Work out the finished part from the listing and answer in its coordinate system (mm). A direction names the side the tool comes from. Give positions to 0.01 mm unless a question says otherwise; leave off trailing zeros. Order: outer loops, then holes, each group sorted by start corner. A loop starts at its lowest first (then second) coordinate and runs counter-clockwise, first axis right, second up. Notation, with made-up numbers: (39.5, 44.25) -> (63.5, 44.25) arc R16 cw to (63.5, 65.25) -> close; hole circle Ø4 at (-19, 84.25). An arc over 180 degrees is marked (long way). Answer as CSV lines item,"result". Start each with the question number.
1. Find the intervals of material crossed by L1, parallel to X at y = 7.2, z = 0; L2, parallel to Z at x = -10.5, y = 13.25; L3, parallel to Y at x = -14.5, z = -18, in increasing order.
2. A cutting plane is placed at A-A (y = 6). Give the vertices of the cut face in (x, z).
3. A cutting plane is placed at B-B (x = 0). Give the vertices of the cut face in (y, z).
4. Flat-ended cylindrical pins translate along their axes: pin 1 (0.7 mm diameter, centred on y = 11.5, z = 3.5, fed in from +X); pin 2 (6 mm diameter, centred on x = -10, y = 17, fed in from -Z); pin 3 (7 mm diameter, centred on x = 0, z = 0, fed in from +Y). Find the tip coordinate at first contact, or state that the pin passes through.
5. A cutting plane is placed at D-D (x = -44). Give the vertices of the cut face in (y, z), then the cut area to 3 significant figures.
6. For faces 1 (the flat face through (-56.2, 18.7, 4.4)), 2 (the flat face through (-64.507, 18.803, -43.287)), 3 (the flat face through (-64, 16, -51.985)), determine the directions among +Z, -Z, +X, -X, +Y, -Y from which every point of the face is accessible in a straight line to the end or side of a thin tool.
7. For a pull along Z with two mould halves and no side action, classify faces 4 (the flat face through (-52.5, 12, 4)), 5 (the flat face through (-56.67, 18.45, 3.29)), 6 (the flat face through (-64, 12, -7.5)) as released by +Z, released by -Z, zero draft, split by the parting line, or undercut.
8. A cutting plane is placed at C-C (z = -56.5). Give the vertices of the cut face in (x, y), then the cut area to 3 significant figures.
from build123d import *

# Parameters (mm, degrees)
SKETCH1_W           = 10.000000000000004
SKETCH1_H           = 10
SKETCH1_W_2         = 10
BOSS_EXTRUDE1_DEPTH = 10
SKETCH2_W           = 1.999999999999993
SKETCH2_H           = 10.29963091051744
SKETCH2_H_2         = 12.500000000000014
BOSS_EXTRUDE2_DEPTH = 12.5
SKETCH3_R           = 1.5000000000000002
SKETCH3_R_2         = 1.5000000000000042
CUT_EXTRUDE1_DEPTH  = 2.200369089
CHAMFER1_SIZE       = 7.5
CHAMFER2_SIZE       = 1
SKETCH4_R           = 1.4999999999999998
SKETCH4_R_2         = 1.5000000000000042
CUT_EXTRUDE2_DEPTH  = 2
CHAMFER3_SIZE       = 7.5
CHAMFER4_SIZE       = 1
CHAMFER5_SIZE       = 1
SKETCH5_R           = 2.6000000000000005
CUT_EXTRUDE3_DEPTH  = 5
CHAMFER6_SIZE       = 1
CHAMFER7_SIZE       = 1
CHAMFER7_SIZE2      = 1.6731571851015008


with BuildPart() as part:
    # Sketch1 → Boss-Extrude1 (new body)
    with BuildSketch(Plane(origin=(0, 0, 0), x_dir=(1, 0, 0), z_dir=(0, 1, 0))):
        Polygon((-12.101007166283637, 51.98463103929535), (-15.740709508945708, 61.984631039295344), (-22.10100716628364, 61.984631039295344), (-22.10100716628364, 51.984631039295344), (-5, 5.000000000000001), (5, 5.000000000000001), align=None)
        with Locations((-27.101007166283644, 56.98463103929535)):
            Rectangle(SKETCH1_W, SKETCH1_H)
        Polygon((-65, 61.984631039295344), (-32.101007166283644, 61.984631039295344), (-32.101007166283644, 51.984631039295344), (-22.10100716628364, 51.984631039295344), (-5, 5.000000000000001), (-5, -5), (-65, -5.000000000000009), align=None)
        Rectangle(SKETCH1_W_2, SKETCH1_H)
    extrude(amount=BOSS_EXTRUDE1_DEPTH)

    # Sketch2 → Boss-Extrude2 (add)
    with BuildSketch(Plane(origin=(0, 10, 0), x_dir=(1, 0, 0), z_dir=(0, 1, 0))):
        with Locations((-64, 2.3501845447412815)):
            Rectangle(SKETCH2_W, SKETCH2_H)
        Polygon((-65, -5.000000000000009), (-63, -5.000000000000007), (-63, -2.799630910517438), (-65, -2.799630910517438), align=None)
        Polygon((-63, -5.000000000000007), (-52.50000000000001, -5), (-52.50000000000001, -2.799630910517438), (-63, -2.799630910517438), align=None)
        Polygon((-17.5, -2.799630910517445), (-17.5, -5), (-5, -5), (-5.000000000000001, -2.799630910517445), align=None)
        with Locations((-64, 45.734631039295344)):
            Rectangle(SKETCH2_W, SKETCH2_H_2)
    extrude(amount=BOSS_EXTRUDE2_DEPTH)

    # Sketch3 → Cut-Extrude1 (cut)
    with BuildSketch(Plane(origin=(0, 0, 2.799630910517438), x_dir=(-1, 0, 0), z_dir=(0, 0, -1))):
        with Locations((10.000000000000002, 15)):
            Circle(SKETCH3_R)
        with Locations((60.00000000000001, 15.000000000000002)):
            Circle(SKETCH3_R_2)
    extrude(amount=-CUT_EXTRUDE1_DEPTH, mode=Mode.SUBTRACT)

    # Chamfer1
    chamfer1_edges = [part.edges().sort_by_distance(p)[0] for p in [
        (-52.50000000000001, 22.5, 3.899815455258719),
        (-17.5, 22.5, 3.8998154552587225),
    ]]
    chamfer(chamfer1_edges, length=CHAMFER1_SIZE)

    # Chamfer2
    chamfer2_edges = [part.edges().sort_by_distance(p)[0] for p in [
        (-56.25000000000001, 18.75, 2.799630910517438),
        (-13.75, 18.75, 2.799630910517445),
    ]]
    chamfer(chamfer2_edges, length=CHAMFER2_SIZE)

    # Sketch4 → Cut-Extrude2 (cut)
    with BuildSketch(Plane(origin=(-63, 0, 0), x_dir=(0, 0, -1), z_dir=(1, 0, 0))):
        with Locations((0, 15)):
            Circle(SKETCH4_R)
        with Locations((47.27277690959397, 15)):
            Circle(SKETCH4_R_2)
    extrude(amount=-CUT_EXTRUDE2_DEPTH, mode=Mode.SUBTRACT)

    # Chamfer3
    chamfer3_edges = [part.edges().sort_by_distance(p)[0] for p in [
        (-64, 22.5, -7.500000000000001),
        (-64, 22.5, -39.48463103929534),
    ]]
    chamfer(chamfer3_edges, length=CHAMFER3_SIZE)

    # Chamfer4
    chamfer4_edges = [part.edges().sort_by_distance(p)[0] for p in [
        (-63, 18.750000000000004, -43.23463103929534),
        (-63, 18.75, -3.750000000000001),
    ]]
    chamfer(chamfer4_edges, length=CHAMFER4_SIZE)

    # Chamfer5
    chamfer5_edges = [part.edges().sort_by_distance(p)[0] for p in [
        (-5.370354754472853, 0, -33.492315519647676),
        (5, 0, 0),
        (-40.37035475447286, 0, -61.984631039295344),
    ]]
    chamfer(chamfer5_edges, length=CHAMFER5_SIZE)

    # Sketch5 → Cut-Extrude3 (cut)
    with BuildSketch(Plane(origin=(0, 10, 0), x_dir=(1, 0, 0), z_dir=(0, 1, 0))):
        with Locations(Location((0, -4.3e-16, 0), (0, 0, 270))):
            Circle(SKETCH5_R)
    extrude(amount=-CUT_EXTRUDE3_DEPTH, mode=Mode.SUBTRACT)

    # Chamfer6
    chamfer6_edges = [part.edges().sort_by_distance(p)[0] for p in [
        (8e-16, 10, -2.6),
    ]]
    chamfer(chamfer6_edges, length=CHAMFER6_SIZE)

    # Chamfer7
    chamfer7_edges = [part.edges().sort_by_distance(p)[0] for p in [
        (-15.740709508945708, 5.5, -61.984631039295344),
    ]]
    chamfer7_side = [part.faces().sort_by_distance(p)[0] for p in [
        (-5.370354754472848, 5.5, -33.49231551964767),
    ]]
    chamfer(chamfer7_edges, length=CHAMFER7_SIZE, length2=CHAMFER7_SIZE2, reference=chamfer7_side[0])


solid = part.part
Answer sheet:
1,L1,"x = -65 to -2.6, 2.6 to 5"
1,L2,"z = 2.8 to 5"
1,L3,"y = 0 to 10"
2,outline,"(-65, -61.98) -> (-17.41, -61.98) -> (-15.4, -61.04) -> (5, -5) -> (5, 5) -> (-65, 5) -> close; hole circle Ø5.2 at (0, 0)"
3,outline,"(0, -15.81) -> (1, -18.74) -> (10, -18.74) -> (10, -3.6) -> (9, -2.6) -> (5, -2.6) -> (5, 2.6) -> (9, 2.6) -> (10, 3.6) -> (10, 5) -> (0, 5) -> close"
4,pin 1,"stops at x = -5"
4,pin 2,"stops at z = 2.8"
4,pin 3,"stops at y = 9.9"
5,outline,"(0, -60.98) -> (1, -61.98) -> (10, -61.98) -> (10, 5) -> (0, 5) -> close"
5,area,"669 mm^2"
6,face 1,"+Z, -Z, +Y"
6,face 2,"+X, -X, +Y"
6,face 3,"-Z, +X, -X, +Y"
7,face 4,"zero draft"
7,face 5,"released by -Z"
7,face 6,"undercut"
8,outline,"(-65, 0) -> (-14.81, 0) -> (-13.74, 1) -> (-13.74, 10) -> (-65, 10) -> close"
8,area,"512 mm^2"
